Input: part model. Units: mm. Frame: model coordinates. Face numbers are marked on the shaded views. A direction names the side the tool comes from. Coordinates: 2 decimals unless noted, no trailing zeros. Write each loop counter-clockwise with the first axis right and the second up, starting at its lowest first coordinate (ties: lowest second). Pieces come first, ordered by that corner, then holes. Notation, with made-up numbers: (67, 86) -> (121, 86) arc R23 cw to (121, 112) -> close; hole circle Ø3 at (-31, -26). An arc over 180 degrees is marked (long way). Use one line per item in the form item = value. Start each with the question number.
(1) Cut plane A-A on x = 0. Return the cut outline in (y, z).
(2) Ray query, line 1 along Z through (x, y) = (0, 0.35); line 2 along Z through (x, y) = (0, 1.6); line 3 along X through (y, z) = (1.5, 0). Return the intervals inside material, ascending.
(3) Set-up query: the marked faces 1 and 2. Return all of +Z, -Z, +X, -X, +Y, -Y with unobstructed straight access to the full face (end or side cutting, diameter ignored); none if empty.
(4) First-contact query: pin 1 (3 mm diameter, centred on x = -11, z = 17.5, fed in from +Y); pin 2 (1.8 mm diameter, centred on x = -20.96, z = 0, fed in from +Y). Flat tips, straight axial feed; report the tip coordinate or a pass-through.
(5) Cut plane B-B on z = -12. Return the cut outline in (x, y), plus the area to 3 significant figures.
(6) Cut plane C-C on x = -9. Return the cut outline in (y, z), plus the area to 3 significant figures.
Autodesk Inventor part; units mm, degrees
ref_plane "YZ Plane" through (0, 0, 0) normal (1, 0, 0) x (0, 1, 0)
ref_plane "XZ Plane" through (0, 0, 0) normal (0, 1, 0) x (-1, 0, 0)
ref_plane "XY Plane" through (0, 0, 0) normal (0, 0, 1) x (1, 0, 0)
sketch "Sketch1" plane through (0, 0, 0) normal (0, 1, 0) x (-1, 0, 0)
  arc A0 (18.9984, 0.2445) -> (18.9984, -0.2445) centre (0, 0) ccw
  circle A1 centre (0, 20.974) radius 0.987
  circle A2 centre (0, -20.974) radius 0.987
  arc A3 (18.9984, 0.2445) -> (18.9984, -0.2445) centre (0, 0) ccw
  arc A4 (18.9984, 0.2445) -> (18.9984, -0.2445) centre (20.9573, 0) ccw
  circle A5 centre (20.9573, 0) radius 0.987
  circle A6 centre (-21.0021, 0) radius 0.987
  arc A7 (-1.4939, 19.6837) -> (-19.6854, 1.4707) centre (0, 0) ccw
  arc A8 (-19.6854, 1.4707) -> (-19.6854, -1.4707) centre (-21.0021, 0) ccw
  arc A9 (-19.6854, -1.4707) -> (-1.4939, -19.6837) centre (0, 0) ccw
  arc A10 (-1.4939, -19.6837) -> (1.4939, -19.6837) centre (0, -20.974) ccw
  arc A11 (1.4939, -19.6837) -> (19.6826, -1.5074) centre (0, 0) ccw
  arc A12 (19.6826, -1.5074) -> (19.6826, 1.5074) centre (20.9573, 0) ccw
  arc A13 (19.6826, 1.5074) -> (1.4939, 19.6837) centre (0, 0) ccw
  arc A14 (1.4939, 19.6837) -> (-1.4939, 19.6837) centre (0, 20.974) ccw
  dimension "d0" = 19
extrude "Extrusion1" add sketch "Sketch1" along normal blind 1
sketch "Sketch2" plane through (0, 1, 0) normal (0, 1, 0) x (1, 0, 0)
  arc A0 (-18.9984, -0.2445) -> (-18.9984, 0.2445) centre (0, 0) ccw
  arc A1 (-18.9984, -0.2445) -> (-18.9984, 0.2445) centre (-20.9573, 0) ccw
  arc A2 (-18.9984, -0.2445) -> (-18.9984, 0.2445) centre (0, 0) ccw
  circle A3 centre (-20.9573, 0) radius 0.987
  circle A4 centre (0, 20.974) radius 0.987
  circle A5 centre (21.0021, 0) radius 0.987
  circle A6 centre (0, -20.974) radius 0.987
  arc A7 (1.4939, -19.6837) -> (19.6854, -1.4707) centre (0, 0) ccw
  arc A8 (19.6854, -1.4707) -> (19.6854, 1.4707) centre (21.0021, 0) ccw
  arc A9 (19.6854, 1.4707) -> (1.4939, 19.6837) centre (0, 0) ccw
  arc A10 (1.4939, 19.6837) -> (-1.4939, 19.6837) centre (0, 20.974) ccw
  arc A11 (-1.4939, 19.6837) -> (-19.6826, 1.5074) centre (0, 0) ccw
  arc A12 (-19.6826, 1.5074) -> (-19.6826, -1.5074) centre (-20.9573, 0) ccw
  arc A13 (-19.6826, -1.5074) -> (-1.4939, -19.6837) centre (0, 0) ccw
  arc A14 (-1.4939, -19.6837) -> (1.4939, -19.6837) centre (0, -20.974) ccw
extrude "Extrusion2" add sketch "Sketch2" along normal mid plane 2 contours A1 A0
sketch "Sketch3" plane through (0, 0, 0) normal (0, -1, 0) x (1, 0, 0)
  point P0 (0, 0)
sketch "Sketch4" plane through (0, 2, 0) normal (0, 1, 0) x (1, 0, 0)
  arc A0 (-18.9984, -0.2445) -> (-18.9984, 0.2445) centre (0, 0) ccw
  circle A1 centre (0, 0) radius 18
  dimension "d5" = 36
extrude "Extrusion3" cut sketch "Sketch4" against normal blind 1
properties part number "tapa"
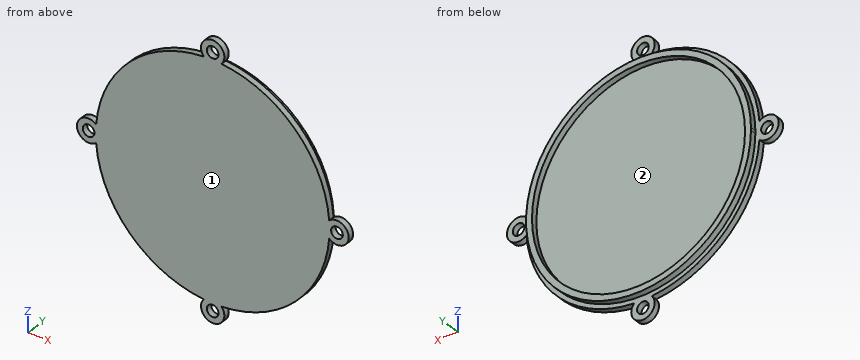
Values:
q1.outline = (0, -22.95) -> (1, -22.95) -> (1, -21.96) -> (0, -21.96) -> close; (0, -19.99) -> (1, -19.99) -> (1, -19) -> (2, -19) -> (2, -18) -> (1, -18) -> (1, 18) -> (2, 18) -> (2, 19) -> (1, 19) -> (1, 19.99) -> (0, 19.99) -> close; (0, 21.96) -> (1, 21.96) -> (1, 22.95) -> (0, 22.95) -> close
q2.line_1 = -22.95 to -21.96, -19.99 to 19.99, 21.96 to 22.95
q2.line_2 = -19 to -18, 18 to 19
q2.line_3 = -18.98 to -18, 18 to 19
q3.face_1 = +Z, -Z, +X, -X, -Y
q3.face_2 = +Y
q4.pin_1 = 1
q4.pin_2 = through
q5.outline = (-15.67, 0) -> (15.67, 0) -> (15.67, 1) -> (14.73, 1) -> (14.73, 2) -> (13.42, 2) -> (13.42, 1) -> (-13.42, 1) -> (-13.42, 2) -> (-14.73, 2) -> (-14.73, 1) -> (-15.67, 1) -> close
q5.area = 34.0 mm2
q6.outline = (0, -17.57) -> (1, -17.57) -> (1, -16.73) -> (2, -16.73) -> (2, -15.59) -> (1, -15.59) -> (1, 15.59) -> (2, 15.59) -> (2, 16.73) -> (1, 16.73) -> (1, 17.57) -> (0, 17.57) -> close
q6.area = 37.4 mm2
